```python
from build123d import *

# Parameters (mm, degrees)
SKETCH2_W          = 14
SKETCH2_H          = 10
CUT_EXTRUDE1_DEPTH = 146
SKETCH3_R          = 8
CUT_EXTRUDE2_DEPTH = 217
CIRPATTERN1_COUNT  = 4


with BuildPart() as part:
    # Sketch1 → Revolve1 (revolve)
    with BuildSketch(Plane(origin=(0, 0, 0), x_dir=(0, 0, -1), z_dir=(1, 0, 0)), mode=Mode.PRIVATE) as revolve1_sk:
        Polygon((-44, 104), (0, 104), (0, 48), (-5, 48), (-5, 25), (-54, 25), (-54, 48), (-24, 48), (-24, 98), (-44, 98), align=None)
    revolve(revolve1_sk.sketch.rotate(Axis((0, 0, 52.496471852), (0, 0, -1)), 90), axis=Axis((0, 0, 52.496471852), (0, 0, -1)))

    # Sketch2 → Cut-Extrude1 (cut)
    with BuildSketch(Plane.XY):
        with Locations((0, 25)):
            Rectangle(SKETCH2_W, SKETCH2_H)
    extrude(amount=CUT_EXTRUDE1_DEPTH, mode=Mode.SUBTRACT)

    # Sketch3 → Cut-Extrude2 (cut)
    with BuildSketch(Plane.XY):
        with Locations(Location((0, 78.704447468, 0), (0, 0, 180))):
            Circle(SKETCH3_R)
    cut_extrude2 = extrude(amount=CUT_EXTRUDE2_DEPTH, mode=Mode.SUBTRACT)

    # CirPattern1: Cut-Extrude2 ×4 about axis
    cirpattern1_axis = Axis((0, 0, 0), (0, 0, 1))
    for i in range(1, CIRPATTERN1_COUNT):
        add(cut_extrude2.rotate(cirpattern1_axis, i * 360 / CIRPATTERN1_COUNT), mode=Mode.SUBTRACT)


solid = part.part
```
Can you work these out from the model? Positions are in its coordinate system, mm. A direction names the side the tool comes from. Give positions to 0.01 mm unless a question says otherwise; leave off trailing zeros. Loops run counter-clockwise (first coordinate to the right, second up) from the corner with the lowest first, then second, coordinate; pieces in that order, holes last. Notation, with made-up numbers: M 62.5,-16 L 72.5,-16 A26 cw 72.5,17 Z; hole C 73.25,27.5 d4. An arc over 180 degrees is marked long. Use CSV: the item, a comma, the result in double quotes. Start each with the question number.
1. Imagine slicing it at C-C, the plane x = 0. Write out the boundary of the cut face in (y, z), plus the area to 3 significant figures.
2. Imagine slicing it at B-B, the plane z = 38.5. Write out the boundary of the cut face in (x, y), plus the area to 3 significant figures.
3. Imagine slicing it at A-A, the plane y = 0. Write out the boundary of the cut face in (x, z).
4. On a 3-axis mill with a long thin cutter (end or side, diameter ignored), from which of +Z, -Z, +X, -X, +Y, -Y can I reach the whole of each face in a straight line? I mean faces 1 (the face through (45, 22, 0)), 2 (the face through (-21, 21, 54)), 3 (the face through (21, 21, 5)), 4 (the face through (-20, -45, 24)), 5 (the face through (0, 30, 29)). Say none if no direction works.
5. Imagine slicing it at D-D, the plane z = 49. Write out the boundary of the cut face in (x, y), plus the area to 3 significant figures.
6. If I drill on L1, parallel to Y at x = 0, z = 21.5; L2, parallel to X at y = -1, z = 32.5; L3, parallel to Y at x = 0, z = 1.25, over which ranges is the centre line in solid material (lowest first)?
7. For P1, Ø8, axis at y = -38, z = 42.5, coming from the -X side; P2, Ø5, axis at y = 26.5, z = 19.5, coming from the -X side; P3, Ø10, axis at y = -47, z = 26, coming from the -X side; P4, Ø2, axis at x = 18.5, y = 14, coming from the +Z side, each with a flat end and sliding along its axis, tell me the tip position at first contact or that it passes through.
8. If we mould it in two halves opening along X, with no side actions, what happens to faces 6 (the face through (70, -70, 44)), 7 (the face through (-1.041, -70.773, 11.832)), 8 (the face through (-82.531, 63.282, 21.692))? For each: released by +X, released by -X, zero draft, split by the parting line, or undercut.
Response values:
1,outline,"M -104,0 L -86.7,0 L -86.7,24 L -98,24 L -98,44 L -104,44 Z; M -70.7,0 L -48,0 L -48,5 L -25,5 L -25,54 L -48,54 L -48,24 L -70.7,24 Z; M 30,5 L 48,5 L 48,0 L 70.7,0 L 70.7,24 L 48,24 L 48,54 L 30,54 Z; M 86.7,0 L 104,0 L 104,44 L 98,44 L 98,24 L 86.7,24 Z"
1,area,"4,170 mm^2"
2,outline,"C 0,0 d208; C 0,0 d96; hole C 0,0 d196; hole M -7,24 A25 ccw long 7,24 L 7,30 L -7,30 Z"
2,area,"9,010 mm^2"
3,outline,"M -104,0 L -86.7,0 L -86.7,24 L -98,24 L -98,44 L -104,44 Z; M -70.7,0 L -48,0 L -48,5 L -25,5 L -25,54 L -48,54 L -48,24 L -70.7,24 Z; M 25,5 L 48,5 L 48,0 L 70.7,0 L 70.7,24 L 48,24 L 48,54 L 25,54 Z; M 86.7,0 L 104,0 L 104,44 L 98,44 L 98,24 L 86.7,24 Z"
4,face 1,"-Z, +X, -X, +Y, -Y"
4,face 2,"+Z, +X, -X, +Y, -Y"
4,face 3,"-Z"
4,face 4,"+Z"
4,face 5,"+Z, -Z"
5,outline,"C 0,0 d96; hole M -7,24 A25 ccw long 7,24 L 7,30 L -7,30 Z"
5,area,"5,200 mm^2"
6,L1,"-104 to -86.7, -70.7 to -25, 30 to 70.7, 86.7 to 104"
6,L2,"-104 to -97.99, -47.99 to -24.98, 24.98 to 47.99, 97.99 to 104"
6,L3,"-104 to -86.7, -70.7 to -48, 48 to 70.7, 86.7 to 104"
7,P1,"x = -98.29"
7,P2,"x = -101.19"
7,P3,"x = -95.14"
7,P4,"through"
8,face 6,"zero draft"
8,face 7,"undercut"
8,face 8,"split by the parting line"
